Verification items for the finished model (mm, model axes). A direction names the side the tool comes from. Round coordinates to 2 decimals unless told otherwise and drop trailing zeros. Order: outer loops, then holes, each group sorted by start corner. A loop starts at its lowest first (then second) coordinate and runs counter-clockwise, first axis right, second up. Notation, with made-up numbers: (11.25, -20.5) -> (48.25, -20.5) arc R14 ccw to (48.25, -7.5) -> close; hole circle Ø7 at (45, 70.25). An arc over 180 degrees is marked (long way). Return JSON: item names as keys, results as strings. Group by question number.
1) Section check B-B on z = -5.5. Enter the section's corners in (x, y).
2) Scan lines: L1, parallel to X at y = 2.5, z = -0.25; L2, parallel to Z at x = 5.5, y = 3; L3, parallel to Y at x = 4.75, z = -9.75. Record each from-to range of solid material in increasing order.
3) Draft check along Z on faces 1 (the cylindrical face through (2.49, 3.45, -6.76)), 2 (the flat face through (2, 0, 0)), 3 (the cylindrical face through (7.55, 3.45, -0.65)), 4 (the cylindrical face through (-0.63, 0.49, 11.56)). Enter one of: pulls with the +Z half, pulls with the -Z half, needs draft (parallel to the pull), parting line crosses it, or undercut.
4) Section check C-C on x = 6.25. Enter the section's corners in (y, z).
5) Tool access check on faces 5 (the cylindrical face through (-4.45, 3.45, -0.65)), 6 (the cylindrical face through (11.418, 3.958, -3.128)). Record the directions out of +Z, -Z, +X, -X, +Y, -Y that give a thin tool (end or side, any length) a straight path to the whole face; none if there is none.
6) Depth check by flat-ended pin: pin 1 (1 mm diameter, centred on y = 4, z = 9.5, fed in from +X); pin 2 (1 mm diameter, centred on x = -7, y = 2.5, fed in from -Z); pin 3 (5.5 mm diameter, centred on x = 0.92, z = -6.26, fed in from +Y); pin 4 (2 mm diameter, centred on x = 9, y = 1.5, fed in from -Z). Enter the tip coordinate at first touch or a pass-through.
7) Section check D-D on z = -0.5. Enter the section's corners in (x, y).
8) Section check A-A on x = 0. Enter the section's corners in (y, z), plus the area to 3 significant figures.
```python
from build123d import *

# Parameters (mm, degrees)
SKETCH1_R           = 9.9
BOSS_EXTRUDE1_DEPTH = 7
SKETCH1_3_R         = 12
BOSS_EXTRUDE2_DEPTH = 1
SKETCH1_4_R         = 1.65
CUT_EXTRUDE1_DEPTH  = 31


with BuildPart() as part:
    # Sketch1 → Boss-Extrude1 (new body)
    with BuildSketch(Plane(origin=(0, 0, 0), x_dir=(1, 0, 0), z_dir=(0, 1, 0))):
        with Locations((1.975062748, 0.154777047)):
            Circle(SKETCH1_R)
    extrude(amount=BOSS_EXTRUDE1_DEPTH)

    # Sketch1<3> → Boss-Extrude2 (add)
    with BuildSketch(Plane(origin=(0, 0, 0), x_dir=(1, 0, 0), z_dir=(0, 1, 0))):
        with Locations((1.975062748, 0.154777047)):
            Circle(SKETCH1_3_R)
    extrude(amount=BOSS_EXTRUDE2_DEPTH)

    # Sketch1<4> → Cut-Extrude1 (cut)
    with BuildSketch(Plane(origin=(0, 0, 0), x_dir=(1, 0, 0), z_dir=(0, 1, 0))):
        with Locations((0.917956723, 6.264264553)):
            Circle(SKETCH1_4_R)
        with Locations((0.917956723, -5.677777134)):
            Circle(SKETCH1_4_R)
        with Locations((-6.024937252, 0.154777047)):
            Circle(SKETCH1_4_R)
        with Locations((5.975062748, 0.154777047)):
            Circle(SKETCH1_4_R)
    extrude(amount=CUT_EXTRUDE1_DEPTH, mode=Mode.SUBTRACT)


solid = part.part
```
Check result:
{
 "1": {"outline": "(-8.77, 0) -> (-0.54, 0) -> (-0.54, 7) -> (-6.36, 7) -> (-6.36, 1) -> (-8.77, 1) -> close; (2.38, 0) -> (12.72, 0) -> (12.72, 1) -> (10.31, 1) -> (10.31, 7) -> (2.38, 7) -> close"},
 "2": {"L1": "-7.92 to -7.67, -4.38 to 4.33, 7.62 to 11.87", "L2": "-9.41 to -1.73, 1.43 to 9.1", "L3": "0 to 1"},
 "3": {"face 1": "undercut", "face 2": "needs draft", "face 3": "undercut", "face 4": "parting line crosses it"},
 "4": {"outline": "(0, -11.37) -> (1, -11.37) -> (1, -9.08) -> (7, -9.08) -> (7, -1.78) -> (0, -1.78) -> close; (0, 1.47) -> (7, 1.47) -> (7, 8.77) -> (1, 8.77) -> (1, 11.06) -> (0, 11.06) -> close"},
 "5": {"face 5": "+Y, -Y", "face 6": "+Y"},
 "6": {"pin 1": "x = 5.74", "pin 2": "z = -5.27", "pin 3": "y = 7", "pin 4": "z = -10.45"},
 "7": {"outline": "(-10.02, 0) -> (-7.64, 0) -> (-7.64, 7) -> (-7.92, 7) -> (-7.92, 1) -> (-10.02, 1) -> close; (-4.41, 0) -> (4.36, 0) -> (4.36, 7) -> (-4.41, 7) -> close; (7.59, 0) -> (13.97, 0) -> (13.97, 1) -> (11.87, 1) -> (11.87, 7) -> (7.59, 7) -> close"},
 "8": {"outline": "(0, -11.99) -> (1, -11.99) -> (1, -9.86) -> (7, -9.86) -> (7, -7.64) -> (0, -7.64) -> close; (0, -4.89) -> (7, -4.89) -> (7, 4.31) -> (0, 4.31) -> close; (0, 7.05) -> (7, 7.05) -> (7, 9.55) -> (1, 9.55) -> (1, 11.68) -> (0, 11.68) -> close", "area": "102 mm^2"}
}
